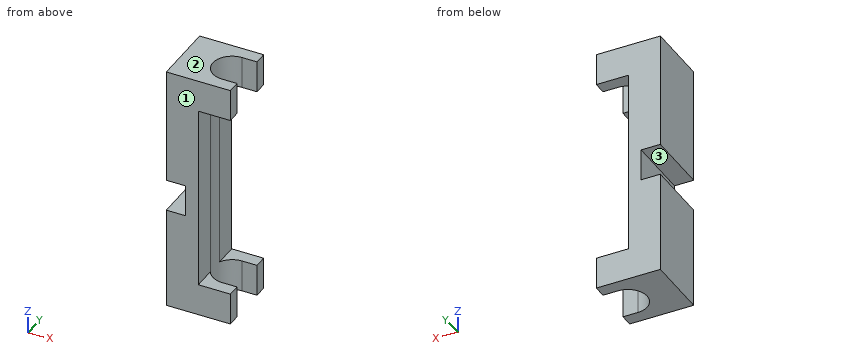
```python
from build123d import *

# Parameters (mm, degrees)
F0_W     = 6.35
F0_H     = 6.35
F1_DEPTH = 12.7
F3_DEPTH = 49.594854
F4_W     = 3.81
F4_H     = 6.35
F5_DEPTH = 25.4


with BuildPart() as f1:
    # F0 (on Front) → F1 (new body)
    with BuildSketch(Plane.XZ):
        Polygon((-21.969653, 32.725027), (-21.969653, -16.868828), (-15.619653, -16.868828), (-15.619653, -10.518828), (-15.619653, 26.375027), (-15.619653, 32.725027), align=None)
        with Locations((-12.444653, -13.693828)):
            Rectangle(F0_W, F0_H)
        with Locations((-12.444653, 29.550027)):
            Rectangle(F0_W, F0_H)
    extrude(amount=F1_DEPTH)

    # F2 (on face) → F3 (cut, through all)
    with BuildSketch(Plane.XY.offset(32.725027)):
        with BuildLine():
            Line((-12.234837, -10.16), (-9.269653, -10.16))
            Line((-9.269653, -10.16), (-9.269653, -2.54))
            Line((-9.269653, -2.54), (-12.234837, -2.54))
            ThreePointArc((-12.234837, -2.54), (-16.044837, -6.35), (-12.234837, -10.16))
        make_face()
    extrude(amount=-F3_DEPTH, mode=Mode.SUBTRACT)

    # F4 (on face) → F5 (cut)
    with BuildSketch(Plane.XZ.offset(12.7)):
        with Locations((-20.064653, 6.530325)):
            Rectangle(F4_W, F4_H)
    extrude(amount=-F5_DEPTH, mode=Mode.SUBTRACT)


solid = f1.part
```
The listing builds one solid part. Answer for the finished solid, in the listing's coordinates (mm). Face numbers are marked on the shaded views. Give positions to 0.01 mm unless a question says otherwise; leave off trailing zeros. Order: outer loops, then holes, each group sorted by start corner. A loop starts at its lowest first (then second) coordinate and runs counter-clockwise, first axis right, second up. Notation, with made-up numbers: (50.5, 27.5) -> (102.5, 27.5) arc R33 cw to (102.5, 57.5) -> close; hole circle Ø10 at (51.5, -20.75). An arc over 180 degrees is marked (long way). One line per item, written item: value.
1) Find section B-B, the plane x = -19. Determine the outline of the cut face in (y, z), plus the area to 3 significant figures.
Reported:
outline: (-12.7, -16.87) -> (0, -16.87) -> (0, 3.36) -> (-12.7, 3.36) -> close; (-12.7, 9.71) -> (0, 9.71) -> (0, 32.73) -> (-12.7, 32.73) -> close
area: 549 mm^2
2) Find section C-C, the plane y = -6.35. Determine the outline of the cut face in (x, z).
Reported:
outline: (-21.97, -16.87) -> (-16.04, -16.87) -> (-16.04, 32.73) -> (-21.97, 32.73) -> (-21.97, 9.71) -> (-18.16, 9.71) -> (-18.16, 3.36) -> (-21.97, 3.36) -> close
3) Flat-ended cylindrical pins translate along their axes: P1, Ø1.4, axis at y = -1.5, z = 2.5, coming from the +X side; P2, Ø1.5, axis at x = -14, z = 12, coming from the +Y side. Find the tip coordinate at first contact, or state that the pin passes through.
Reported:
P1: stops at x = -15.62
P2: passes through
4) Find the intervals of material crossed by line 1 (Z direction, x = -21, y = -2.25); line 2 (Z direction, x = -10.75, y = -1); line 3 (Y direction, x = -11.5, z = 27), in increasing order.
Reported:
line 1: z = -16.87 to 3.36, 9.71 to 32.73
line 2: z = -16.87 to -10.52, 26.38 to 32.73
line 3: y = -12.7 to -10.16, -2.54 to 0
5) Find section A-A, the plane x = -10. Determine the outline of the cut face in (y, z).
Reported:
outline: (-12.7, -16.87) -> (-10.16, -16.87) -> (-10.16, -10.52) -> (-12.7, -10.52) -> close; (-12.7, 26.38) -> (-10.16, 26.38) -> (-10.16, 32.73) -> (-12.7, 32.73) -> close; (-2.54, -16.87) -> (0, -16.87) -> (0, -10.52) -> (-2.54, -10.52) -> close; (-2.54, 26.38) -> (0, 26.38) -> (0, 32.73) -> (-2.54, 32.73) -> close
6) Determine the mould class of the marked faces 1, 2 and 3 for opening direction Z: pulls with the +Z half, pulls with the -Z half, needs draft (parallel to the pull), parting line crosses it, or undercut.
Reported:
face 1: needs draft
face 2: pulls with the +Z half
face 3: undercut
7) Find section D-D, the plane z = 6.5. Determine the outline of the cut face in (x, y), plus the area to 3 significant figures.
Reported:
outline: (-18.16, -12.7) -> (-15.62, -12.7) -> (-15.62, -8.1) arc R3.81 cw to (-15.62, -4.6) -> (-15.62, 0) -> (-18.16, 0) -> close
area: 31.3 mm^2
